The model under review builds one solid part; all positions refer to its coordinate system, in mm. A direction names the side the tool comes from. Coordinates: 2 decimals unless noted, no trailing zeros. Loops run counter-clockwise (first coordinate to the right, second up) from the corner with the lowest first, then second, coordinate; pieces in that order, holes last. Notation, with made-up numbers: M -33,38.25 L -16,38.25 A24 cw -16,52.25 Z; hole C 5,43.25 d8. An arc over 180 degrees is marked long. One line per item, written item: value.
```python
from build123d import *

# Parameters (mm, degrees)
F1_DEPTH  = 15
F2_R      = 5.9679112776
F3_DEPTH  = 5.2
F7_R      = 5.9679112776
F6_R      = 5.9679112776
F5_R      = 5.9679112776
F4_R      = 5.9679112776
F8_R      = 5.9679112776
F9_DEPTH  = 5.2
F10_R     = 5.9679112776
F11_R     = 5.9679112776
F12_DEPTH = 5.2
F13_R     = 0.5008771255
F14_DEPTH = 25


with BuildPart() as f1:
    # F0 (on Top) → F1 (new body)
    with BuildSketch(Plane.XY):
        Polygon((0, -28.6071354192), (24.7745060026, -14.3035677096), (24.7745060026, 14.3035677096), (0, 28.6071354192), (-24.7745060026, 14.3035677096), (-24.7745060026, -14.3035677096), align=None)
    extrude(amount=F1_DEPTH)

    # F2 (on face) → F3 (cut)
    with BuildSketch(Plane(origin=(-12.3872530013, 21.4553515644, 0), x_dir=(-0.8660254038, -0.5, 0), z_dir=(-0.5, 0.8660254038, 0))):
        with Locations((0, 7.6934061944)):
            Circle(F2_R)
    extrude(amount=-F3_DEPTH, mode=Mode.SUBTRACT)

    # F7 (on face) + F6 (on face) + F5 (on face) + F4 (on face) + F8 (on face) → F9 (cut)
    with BuildSketch(Plane.YZ.offset(24.7745060026)):
        with Locations((0, 7.5)):
            Circle(F7_R)
    with BuildSketch(Plane(origin=(12.3872530013, -21.4553515644, 0), x_dir=(0.8660254038, 0.5, 0), z_dir=(0.5, -0.8660254038, 0))):
        with Locations((0, 7.5)):
            Circle(F6_R)
    with BuildSketch(Plane(origin=(-12.3872530013, -21.4553515644, 0), x_dir=(0.8660254038, -0.5, 0), z_dir=(-0.5, -0.8660254038, 0))):
        with Locations((0, 7.5)):
            Circle(F5_R)
    with BuildSketch(Plane(origin=(-24.7745060026, 0, 0), x_dir=(0, -1, 0), z_dir=(-1, 0, 0))):
        with Locations((0, 7.5)):
            Circle(F4_R)
    with BuildSketch(Plane(origin=(12.3872530013, 21.4553515644, 0), x_dir=(-0.8660254038, 0.5, 0), z_dir=(0.5, 0.8660254038, 0))):
        with Locations((0, 7.5)):
            Circle(F8_R)
    extrude(amount=-F9_DEPTH, dir=(1, 0, 0), mode=Mode.SUBTRACT)

    # F10 (on face) + F11 (on face) → F12 (cut)
    with BuildSketch(Plane(origin=(-24.7745060026, 0, 0), x_dir=(0, -1, 0), z_dir=(-1, 0, 0))):
        with Locations((0, 7.5)):
            Circle(F10_R)
    with BuildSketch(Plane(origin=(-12.3872530013, -21.4553515644, 0), x_dir=(0.8660254038, -0.5, 0), z_dir=(-0.5, -0.8660254038, 0))):
        with Locations((0, 7.5)):
            Circle(F11_R)
    extrude(amount=-F12_DEPTH, dir=(-1, 0, 0), mode=Mode.SUBTRACT)

    # F13 (on face) → F14 (cut)
    with BuildSketch(Plane.XY.offset(15)):
        Circle(F13_R)
    extrude(amount=-F14_DEPTH, mode=Mode.SUBTRACT)


solid = f1.part
```
(1) Insertion check: pin 1 Ø0.8 at (x, y) = (0, 0) entering from +Z; pin 2 Ø3.5 at (y, z) = (-1, 7.5) entering from -X; pin 3 Ø3 at (x, z) = (-7.5, 2) entering from +Y; pin 4 Ø7 at (y, z) = (0, 7.5) entering from +X. Each pin has a flat end and moves straight along its axis. Give the tip position at first contact, or say it passes through.
Checks:
pin 1: through
pin 2: x = -19.57
pin 3: y = 25.14
pin 4: x = 19.57
(2) Add section B-B on x = 4. State how many separate pieces and enclosed holes the cut face has, then the cut area to 3 significant figures.
Checks:
separate pieces: 1
enclosed holes: 2
area: 774 mm^2
(3) Add section A-A on x = -18.5. State the section outline as (y, z) points.
Checks:
outline: M -17.93,0 L 17.93,0 L 17.93,15 L -17.93,15 Z
(4) Draft analysis for pull direction Y (two halves, no side actions). For faces 5 (the face through (0, -6, 15)), 6 (the face through (7.26, 21.414, 7.584)), 7 (the face through (6.708, -24.734, 7.395)), state which applies: pulls with the +Y half, pulls with the -Y half, needs draft (parallel to the pull), parting line crosses it, or undercut.
Checks:
face 5: needs draft
face 6: undercut
face 7: pulls with the -Y half
(5) To check wall thickness, follow L1, parallel to Z at x = 21.9, y = 0; L2, parallel to Y at x = 10.5, z = 13.25; L3, parallel to Y at x = 0, z = 8.75. State the ranges of each line that lie inside material, in increasing order. Write a range as [from, to].
Checks:
L1: [0, 1.53], [13.47, 15]
L2: [-22.54, -22.25], [-20.66, 20.66], [22.25, 22.54]
L3: [-28.61, -0.5], [0.5, 28.61]
(6) Tool access review of faces 1 (the face through (19.575, 0, 8)), 2 (the face through (-9.715, 16.994, 7.777)), 3 (the face through (-19.575, 0, 8)), 4 (the face through (-24.775, 3, 2)): name each direction out of +Z, -Z, +X, -X, +Y, -Y from which nothing blocks a thin tool from reaching the whole face with its end or side.
Checks:
face 1: +X
face 2: none
face 3: -X
face 4: +Z, -Z, -X, +Y, -Y
